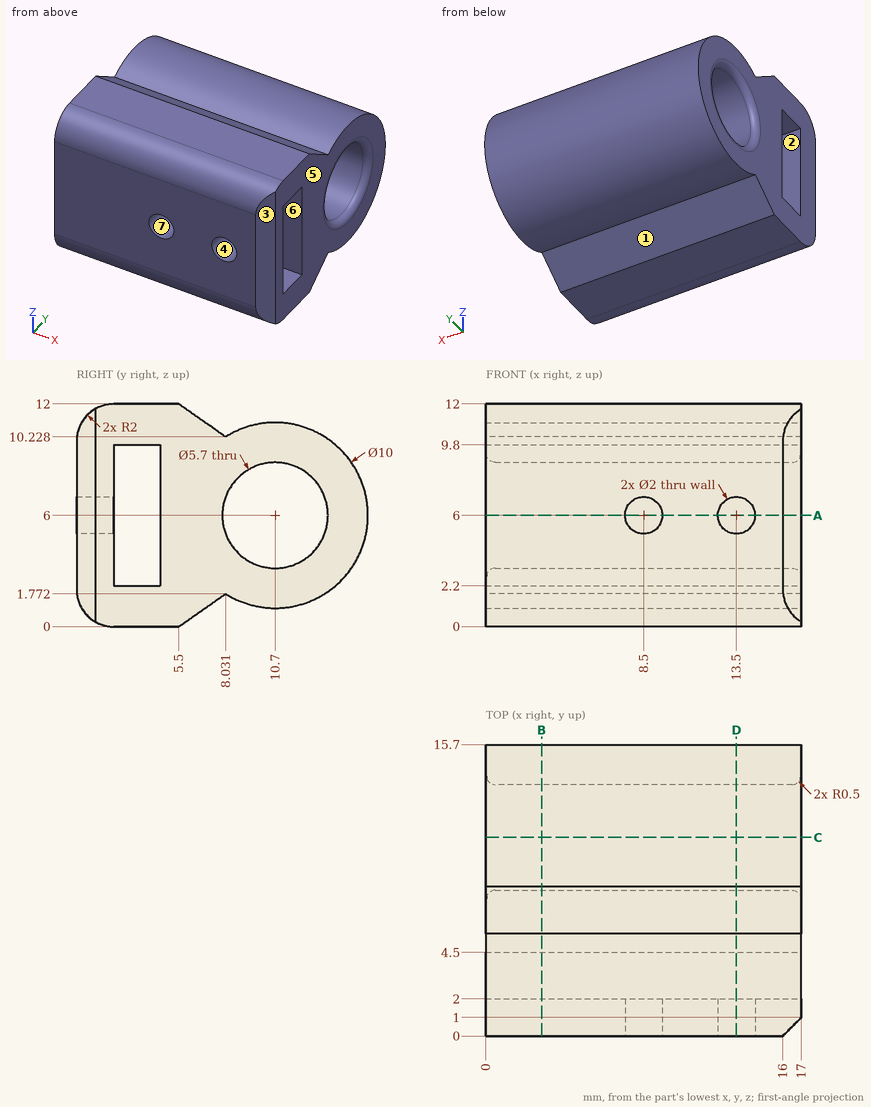
The figure shows three views and two pictorial views of one solid part (mm, origin at its lowest corner). Answer the questions. A direction names the side the tool comes from. Round coordinates to 2 decimals unless told otherwise and drop trailing zeros. Order: outer loops, then holes, each group sorted by start corner. A loop starts at its lowest first (then second) coordinate and runs counter-clockwise, first axis right, second up. Notation, with made-up numbers: (75.25, 76) -> (131.25, 76) arc R12 ccw to (131.25, 85) -> close; hole circle Ø6 at (40.5, 21.5). An arc over 180 degrees is marked (long way). Put each result on its own line as item: value.
Q1. Section A-A, the plane z = 6 is taken. Write down the section's boundary in (x, y).
Results list:
outline: (0, 0) -> (7.5, 0) -> (7.5, 2) -> (0, 2) -> close; (0, 4.5) -> (17, 4.5) -> (17, 7.35) arc R0.5 ccw to (16.5, 7.85) -> (0.5, 7.85) arc R0.5 ccw to (0, 7.35) -> close; (0, 14.05) arc R0.5 ccw to (0.5, 13.55) -> (16.5, 13.55) arc R0.5 ccw to (17, 14.05) -> (17, 15.7) -> (0, 15.7) -> close; (9.5, 0) -> (12.5, 0) -> (12.5, 2) -> (9.5, 2) -> close; (14.5, 0) -> (16, 0) -> (17, 1) -> (17, 2) -> (14.5, 2) -> close
Q2. Section B-B, the plane x = 3 is taken. Write down the section's boundary in (y, z), and give its area (3 significant figures).
Results list:
outline: (0, 2) arc R2 ccw to (2, 0) -> (5.5, 0) -> (8.03, 1.77) arc R5 ccw (long way) to (8.03, 10.23) -> (5.5, 12) -> (2, 12) arc R2 ccw to (0, 10) -> close; hole (2, 2.2) -> (4.5, 2.2) -> (4.5, 9.8) -> (2, 9.8) -> close; hole circle Ø5.7 at (10.7, 6)
area: 110 mm^2
Q3. Which of the six approach directions +Z, -Z, +X, -X, +Y, -Y give full straight-line access (tool end or side, diameter ignored) to the marked faces 1, 2 and 3?
Results list:
face 1: -Z, +X, -X
face 2: +X, -X
face 3: +Z, -Z, +X, -Y
Q4. Determine the mould class of the marked faces 4, 5, 6 and 7 for opening direction X: pulls with the +X half, pulls with the -X half, needs draft (parallel to the pull), parting line crosses it, or undercut.
Results list:
face 4: undercut
face 5: pulls with the +X half
face 6: needs draft
face 7: undercut
Q5. Each of these flat-tipped pins is pushed along its axis until it touches: P1, Ø6, axis at x = 10, z = 4.5, coming from the +Y side; P2, Ø4, axis at x = 2.5, z = 2.5, coming from the +Y side; P3, Ø3.5, axis at y = 10.7, z = 6, coming from the +X side (3 decimals); P4, Ø1, axis at x = 11.5, y = 12.5, coming from the +Z side. Where does it stop, or does it pass through?
Results list:
P1: y = 15.7
P2: y = 15.47
P3: through
P4: z = 10.83
Q6. Section C-C, the plane y = 10.7 is taken. Write down the section's boundary in (x, z).
Results list:
outline: (0, 1) -> (17, 1) -> (17, 2.65) arc R0.5 ccw to (16.5, 3.15) -> (0.5, 3.15) arc R0.5 ccw to (0, 2.65) -> close; (0, 9.35) arc R0.5 ccw to (0.5, 8.85) -> (16.5, 8.85) arc R0.5 ccw to (17, 9.35) -> (17, 11) -> (0, 11) -> close
Q7. Consider line 1 along X through (y, z) = (1.45, 6); line 2 along Z through (x, y) = (13, 10.7); line 3 along Y through (x, z) = (5, 8). Determine where each line is inside the solid, lowest interval first.
Results list:
line 1: 0 to 7.5, 9.5 to 12.5, 14.5 to 17
line 2: 1 to 3.15, 8.85 to 11
line 3: 0 to 2, 4.5 to 8.67, 12.73 to 15.28
Q8. Section D-D, the plane x = 13.5 is taken. Write down the section's boundary in (y, z).
Results list:
outline: (0, 2) arc R2 ccw to (2, 0) -> (5.5, 0) -> (8.03, 1.77) arc R5 ccw (long way) to (8.03, 10.23) -> (5.5, 12) -> (2, 12) arc R2 ccw to (0, 10) -> (0, 7) -> (2, 7) -> (2, 9.8) -> (4.5, 9.8) -> (4.5, 2.2) -> (2, 2.2) -> (2, 5) -> (0, 5) -> close; hole circle Ø5.7 at (10.7, 6)
